Study the drawing (mm; zero at the part's minimum x, y, z) and answer. Coordinates: 2 decimals unless noted, no trailing zeros. Loops run counter-clockwise (first coordinate to the right, second up) from the corner with the lowest first, then second, coordinate; pieces in that order, holes last. Notation, with made-up numbers: (51.5, 63) - (98.5, 63) arc R22 cw to (98.5, 96) - close; hole circle Ø6 at (8, 7). An arc over 180 degrees is marked (long way). Use one line per item in the form item = value.
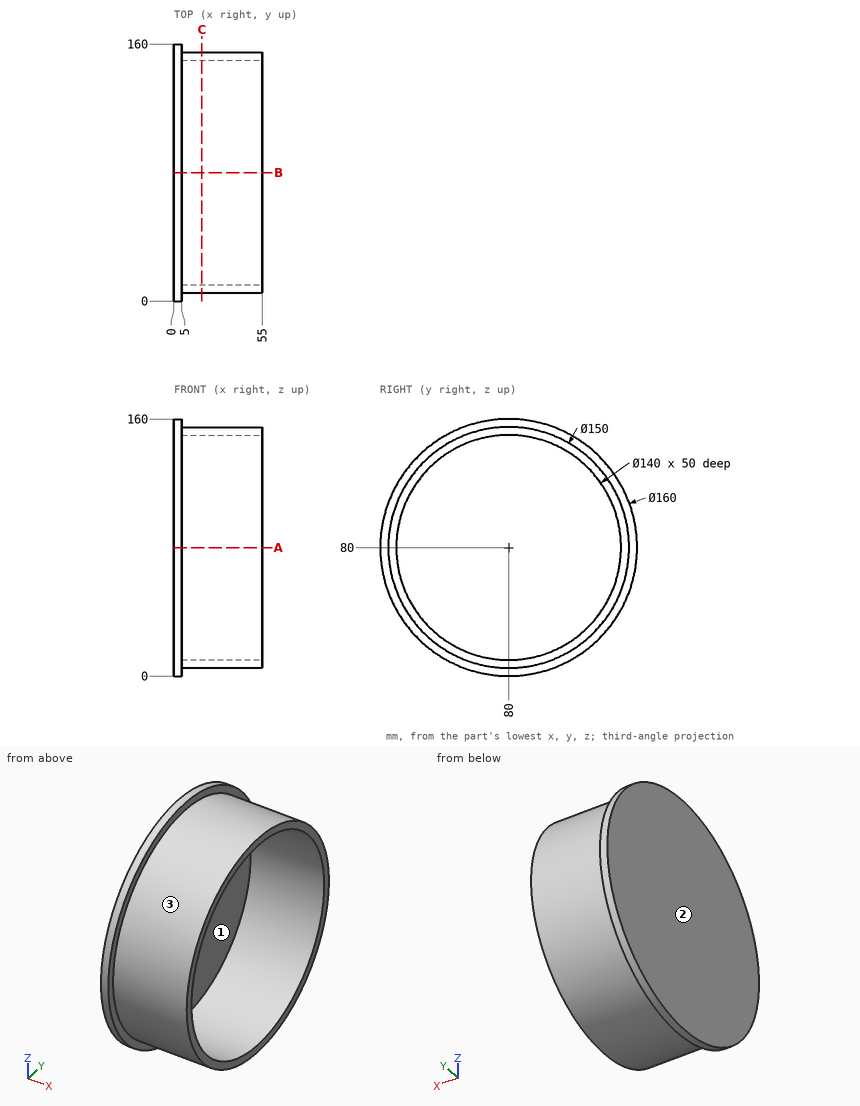
Item 1: The part is cut by section C-C on x = 17.5. Give the vertices of the cut face in (y, z).
Results below:
outline = circle Ø150 at (80, 80); hole circle Ø140 at (80, 80)
Item 2: Find the intervals of material crossed by L1, parallel to Y at x = 16, z = 80; L2, parallel to X at y = 32, z = 47.5; L3, parallel to Y at x = 21, z = 34.5, in increasing order.
Results below:
L1 = 5 to 10, 150 to 155
L2 = 0 to 5
L3 = 20.38 to 26.8, 133.2 to 139.62
Item 3: For a pull along Y with two mould halves and no side action, classify the marked faces 1, 2 and 3 as +Y half, -Y half, draft (parallel to the pull), parting line (faces both ways), or undercut.
Results below:
face_1 = undercut
face_2 = draft
face_3 = parting line
Item 4: The part is cut by section A-A on z = 80. Give the vertices of the cut face in (x, y).
Results below:
outline = (0, 0) - (5, 0) - (5, 5) - (55, 5) - (55, 10) - (5, 10) - (5, 150) - (55, 150) - (55, 155) - (5, 155) - (5, 160) - (0, 160) - close
Item 5: Each of these flat-tipped pins is pushed along its axis until it touches: P1, Ø8, axis at y = 106, z = 45.5, coming from the +X side; P2, Ø1.5, axis at x = 46, y = 101, coming from the +Z side; P3, Ø2, axis at x = 36, y = 66.5, coming from the -Z side. Where does it stop, or does it pass through?
Results below:
P1 = 5
P2 = 152.21
P3 = 6.05
